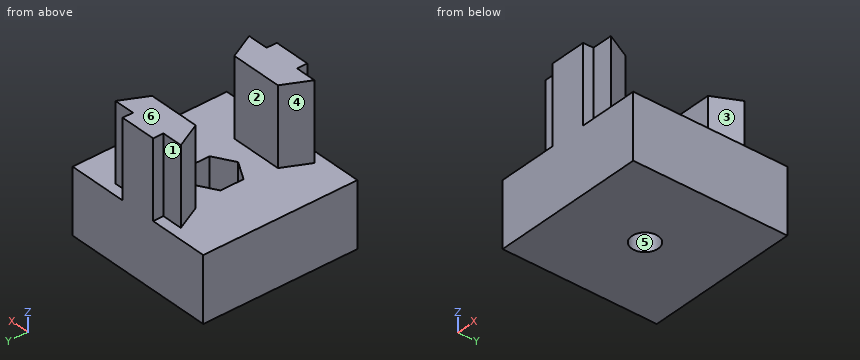
Autodesk Fusion 360 part; units mm, degrees
sketch "Sketch1" plane through (0, 0, 0) normal (0, 0, 1) x (1, 0, 0)
  line L0 (0, 0) -> (30, 0)
  line L1 (30, 0) -> (30, 30)
  line L2 (30, 30) -> (0, 30)
  line L3 (0, 30) -> (0, 0)
  dimension "d1" = 30
  dimension "d2" = 30
extrude "Extrude1" add sketch "Sketch1" along normal blind 12.5
sketch "Sketch2" plane through (0, 0, 12.5) normal (0, 0, 1) x (-1, 0, 0)
  line L0 (0, -30) -> (0, 0)
  line L1 (0, 0) -> (-30, 0)
  line L2 (-30, 0) -> (-30, -30)
  line L3 (-30, -30) -> (0, -30)
  line L4 (-15, -30) -> (-11.5, -30)
  line L5 (-15, -30) -> (-18.5, -30)
  line L6 (-18.5, -30) -> (-18.5, -28)
  line L7 (-11.5, -30) -> (-11.5, -28)
  line L8 (-15, -28) -> (-22.5, -28)
  line L9 (-15, -28) -> (-7.5, -28)
  line L10 (-15, -30) -> (-15, -23)
  line L11 (-15, -23) -> (-10, -23)
  line L12 (-15, -23) -> (-20, -23)
  line L13 (-10, -23) -> (-7.5, -28)
  line L14 (-20, -23) -> (-22.5, -28)
  dimension "d5" = 3.5
  dimension "d6" = 3.5
  dimension "d7" = 7.5
  dimension "d8" = 7.5
  dimension "d9" = 7
  dimension "d10" = 5
  dimension "d11" = 5
extrude "Extrude2" add sketch "Sketch2" along normal blind 15 contours L3 L4 L7 L9 L10 | L3 L5 L6 L8 L10 | L9 L10 L11 L13 | L8 L10 L12 L14
sketch "Sketch3" plane through (0, 0, 12.5) normal (0, 0, 1) x (-1, 0, 0)
  line L0 (-18.5, -30) -> (-18.5, -28)
  line L1 (-18.5, -28) -> (-22.5, -28)
  line L2 (-22.5, -28) -> (-20, -23)
  line L3 (-20, -23) -> (-10, -23)
  line L4 (-10, -23) -> (-7.5, -28)
  line L5 (-7.5, -28) -> (-11.5, -28)
  line L6 (-11.5, -28) -> (-11.5, -30)
  line L7 (-11.5, -30) -> (0, -30)
  line L8 (0, -30) -> (0, 0)
  line L9 (0, 0) -> (-30, 0)
  line L10 (-30, 0) -> (-30, -30)
  line L11 (-30, -30) -> (-18.5, -30)
  line L12 (-11.5, 0) -> (-11.5, -2)
  line L13 (-18.5, 0) -> (-18.5, -2)
  line L14 (-11.5, -2) -> (-7.5, -2)
  line L15 (-18.5, -2) -> (-22.5, -2)
  line L16 (-15, 0) -> (-15, -7)
  line L17 (-15, -7) -> (-20, -7)
  line L18 (-20, -7) -> (-22.5, -2)
  line L19 (-15, -7) -> (-10, -7)
  line L20 (-7.5, -2) -> (-10, -7)
  dimension "d15" = 4
  dimension "d16" = 4
  dimension "d17" = 7
  dimension "d18" = 5
extrude "Extrude3" add sketch "Sketch3" along normal blind 15 contours L9 L13 L15 L16 L17 L18 | L9 L12 L14 L16 L19 L20
sketch "Sketch4" plane through (0, 0, 12.5) normal (0, 0, 1) x (-1, 0, 0)
  line L0 (-18.5, -2) -> (-18.5, 0)
  line L1 (-18.5, 0) -> (-30, 0)
  line L2 (-30, 0) -> (-30, -30)
  line L3 (-30, -30) -> (-18.5, -30)
  line L4 (-18.5, -30) -> (-18.5, -28)
  line L5 (-18.5, -28) -> (-22.5, -28)
  line L6 (-22.5, -28) -> (-20, -23)
  line L7 (-20, -23) -> (-10, -23)
  line L8 (-10, -23) -> (-7.5, -28)
  line L9 (-7.5, -28) -> (-11.5, -28)
  line L10 (-11.5, -28) -> (-11.5, -30)
  line L11 (-11.5, -30) -> (0, -30)
  line L12 (0, -30) -> (0, 0)
  line L13 (0, 0) -> (-11.5, 0)
  line L14 (-11.5, 0) -> (-11.5, -2)
  line L15 (-11.5, -2) -> (-7.5, -2)
  line L16 (-7.5, -2) -> (-10, -7)
  line L17 (-10, -7) -> (-20, -7)
  line L18 (-20, -7) -> (-22.5, -2)
  line L19 (-22.5, -2) -> (-18.5, -2)
  line L20 (-15, -10.5) -> (-18.8971, -12.75)
  line L21 (-18.8971, -12.75) -> (-18.8971, -17.25)
  line L22 (-18.8971, -17.25) -> (-15, -19.5)
  line L23 (-15, -19.5) -> (-11.1029, -17.25)
  line L24 (-11.1029, -17.25) -> (-11.1029, -12.75)
  line L25 (-11.1029, -12.75) -> (-15, -10.5)
  point P0 (-15, -15)
  dimension "d21" = 4.5
extrude "Extrude4" cut sketch "Sketch4" against normal blind 6 contours L20 L21 L22 L23 L24 L25
sketch "Sketch5" plane through (0, 0, 6.5) normal (0, 0, 1) x (-1, 0, 0)
  line L0 (-11.1029, -12.75) -> (-15, -10.5)
  line L1 (-15, -10.5) -> (-18.8971, -12.75)
  line L2 (-18.8971, -12.75) -> (-18.8971, -17.25)
  line L3 (-18.8971, -17.25) -> (-15, -19.5)
  line L4 (-15, -19.5) -> (-11.1029, -17.25)
  line L5 (-11.1029, -17.25) -> (-11.1029, -12.75)
  circle A0 centre (-15, -15) radius 2.55
  dimension "d24" = 5.1
extrude "Extrude5" cut sketch "Sketch5" against normal blind 50 contours A0
equation "d7 = ( 15 / 2 ) * 1 mm"
equation "d21 = ( 9 / 2 ) * 1 mm"
Design review of the part built by this model. Coordinates are the model's own, in mm. Face numbers are marked on the shaded views. A direction names the side the tool comes from. Coordinates: 2 decimals unless noted, no trailing zeros. Loops run counter-clockwise (first coordinate to the right, second up) from the corner with the lowest first, then second, coordinate; pieces in that order, holes last. Notation, with made-up numbers: (57.25, 65) -> (94.25, 65) arc R28 ccw to (94.25, 97) -> close; hole circle Ø2 at (-24.75, 75.25). An arc over 180 degrees is marked (long way). Use a Markdown table: item, result. Add a question column.
Item 1: The part is to be moulded in two halves that separate along X. For the marked faces 4, 5 and 6, say which applies: +X half, -X half, draft (parallel to the pull), parting line (faces both ways), or undercut.
Item 2: Clearance check with flat-ended pins moving along their axes: P1, Ø6, axis at y = 3.5, z = 19, coming from the +X side; P2, Ø8, axis at x = 10, z = 22, coming from the +Y side; P3, Ø0.6, axis at y = 1, z = 19.5, coming from the -X side; P4, Ø2, axis at x = 10, z = 22.5, coming from the -Y side. State where each tip first meets the part, or that it passes through.
Item 3: We need section D-D, the plane x = 20.75. Write out the cut boundary in (y, z), and give its area (3 significant figures).
Item 4: We need section C-C, the plane z = 8.5. Write out the cut boundary in (x, y).
Item 5: We need section B-B, the plane y = 15. Write out the cut boundary in (x, z), and give its area (3 significant figures).
Item 6: Wall thickness on L1, parallel to X at y = 15, z = 4.25; L2, parallel to Y at x = 15.75, z = 13: over which ranges is each line inside the solid? List them lowest first. Write a range as from..to.
Item 7: Machinability: for the marked faces 1, 2 and 3, which of the approach directions +Z, -Z, +X, -X, +Y, -Y give a long, thin tool a straight path to every point of the face, cutting with its end or side? Answer none if there is none.
Item 8: We need section A-A, the plane z = 20.25. Write out the cut boundary in (x, y), and give its area (3 significant figures).
Numbers:
| question | item | result |
|---|---|---|
| 1 | face 4 | -X half |
| 1 | face 5 | undercut |
| 1 | face 6 | draft |
| 2 | P1 | stops at x = 22.5 |
| 2 | P2 | stops at y = 30 |
| 2 | P3 | stops at x = 11.5 |
| 2 | P4 | stops at y = 2 |
| 3 | outline | (0, 0) -> (30, 0) -> (30, 12.5) -> (28, 12.5) -> (28, 27.5) -> (24.5, 27.5) -> (24.5, 12.5) -> (5.5, 12.5) -> (5.5, 27.5) -> (2, 27.5) -> (2, 12.5) -> (0, 12.5) -> close |
| 3 | area | 480 mm^2 |
| 4 | outline | (0, 0) -> (30, 0) -> (30, 30) -> (0, 30) -> close; hole (11.1, 12.75) -> (15, 10.5) -> (18.9, 12.75) -> (18.9, 17.25) -> (15, 19.5) -> (11.1, 17.25) -> close |
| 5 | outline | (0, 0) -> (12.45, 0) -> (12.45, 6.5) -> (11.1, 6.5) -> (11.1, 12.5) -> (0, 12.5) -> close; (17.55, 0) -> (30, 0) -> (30, 12.5) -> (18.9, 12.5) -> (18.9, 6.5) -> (17.55, 6.5) -> close |
| 5 | area | 295 mm^2 |
| 6 | L1 | x = 0..12.45, 17.55..30 |
| 6 | L2 | y = 0..7, 23..30 |
| 7 | face 1 | +Z, -X, +Y |
| 7 | face 2 | +Z, +X, -X |
| 7 | face 3 | +Z, +X |
| 8 | outline | (7.5, 2) -> (11.5, 2) -> (11.5, 0) -> (18.5, 0) -> (18.5, 2) -> (22.5, 2) -> (20, 7) -> (10, 7) -> close; (7.5, 28) -> (10, 23) -> (20, 23) -> (22.5, 28) -> (18.5, 28) -> (18.5, 30) -> (11.5, 30) -> (11.5, 28) -> close |
| 8 | area | 153 mm^2 |
